```python
from build123d import *

# Parameters (mm, degrees)
IZIM1_R                     = 4.2
Y_KSEKLIK_EKSTR_ZYON1_DEPTH = 12
Y_KSEKLIK_EKSTR_ZYON2_DEPTH = 48
Y_KSEKLIK_EKSTR_ZYON3_DEPTH = 3.5


with BuildPart() as part:
    # Çizim1 → Yükseklik-Ekstrüzyon1 (new body)
    with BuildSketch(Plane.XY):
        with BuildLine():
            Line((-17.5, 16), (17.5, 16))
            ThreePointArc((17.5, 16), (24.571067812, 13.071067812), (27.5, 6))
            Line((27.5, 6), (27.5, -16))
            Line((27.5, -16), (-27.5, -16))
            Line((-27.5, -16), (-27.5, 6))
            ThreePointArc((-27.5, 6), (-24.571067812, 13.071067812), (-17.5, 16))
        make_face()
        with Locations((-20, 6)):
            Circle(IZIM1_R, mode=Mode.SUBTRACT)
        with Locations((20, 6)):
            Circle(IZIM1_R, mode=Mode.SUBTRACT)
    extrude(amount=Y_KSEKLIK_EKSTR_ZYON1_DEPTH)

    # Çizim2 → Yükseklik-Ekstrüzyon2 (add)
    with BuildSketch(Plane.XY.offset(12)):
        with BuildLine():
            Line((-27.5, -16), (-12, -16))
            Line((-12, -16), (-12, -8))
            Line((-12, -8), (12, -8))
            Line((12, -8), (12, -16))
            Line((12, -16), (27.5, -16))
            Line((27.5, -16), (27.5, -4))
            ThreePointArc((27.5, -4), (26.328427125, -1.171572875), (23.5, 0))
            Line((23.5, 0), (-23.5, 0))
            ThreePointArc((-23.5, 0), (-26.328427125, -1.171572875), (-27.5, -4))
            Line((-27.5, -4), (-27.5, -16))
        make_face()
    extrude(amount=Y_KSEKLIK_EKSTR_ZYON2_DEPTH)

    # Çizim3 → Yükseklik-Ekstrüzyon3 (add, symmetric)
    with BuildSketch(Plane(origin=(0, 0, 0), x_dir=(0, 0, -1), z_dir=(1, 0, 0))):
        Polygon((-12, 16), (-47, 0), (-12, 0), align=None)
    extrude(amount=Y_KSEKLIK_EKSTR_ZYON3_DEPTH, both=True)


solid = part.part
```
Can you work these out from the model? Positions are in its coordinate system, mm. A direction names the side the tool comes from. Round coordinates to 2 decimals unless told otherwise and drop trailing zeros. Loops run counter-clockwise (first coordinate to the right, second up) from the corner with the lowest first, then second, coordinate; pieces in that order, holes last. Notation, with made-up numbers: M -4.5,-39.75 L -0.5,-39.75 A22 ccw -0.5,-16.75 Z; hole C 1,52.25 d8. An arc over 180 degrees is marked long. Answer as a JSON object with one key per item and string values. Group by question number.
Q1. Will these pins go through, and if not, where does the flat tip stop? pin 1 (17.5 mm diameter, centred on y = 9.5, z = 30.5, fed in from -X); pin 2 (5 mm diameter, centred on y = 8.5, z = 24.5, fed in from +X); pin 3 (12 mm diameter, centred on y = 3, z = 52.5, fed in from -X); pin 4 (5 mm diameter, centred on x = 20, y = 6, fed in from +Z).
Q2. Please list where these lines run through material, in increasing order: L1, parallel to Z at x = 1.5, y = -9; L2, parallel to Y at x = 20, z = 4; L3, parallel to Y at x = -8, z = 12.5.
Q3. On a 3-axis mill with a long thin cutter (end or side, diameter ignored), from which of +Z, -Z, +X, -X, +Y, -Y can I reach the whole of each face in a straight line? I mean faces 4 (the flat face through (3.5, 5, 22)), 5 (the flat face through (6, 0, 36)), 6 (the flat face through (-15, 8, 12)), 7 (the flat face through (-12, -12, 36)). Say none if no direction works.
Q4. Imagine slicing it at B-B, the plane x = -20. Please give me the cut outline in (y, z), then the cut area to 3 significant figures.
Q5. Imagine slicing it at A-A, the plane z = 6.5. Please give me the cut outline in (x, y).
Q6. Imagine slicing it at C-C, the plane z = 26. Please give me the cut outline in (x, y), then the cut area to 3 significant figures.
Q7. Imagine slicing it at D-D, the plane y = -2. Please give me the cut outline in (x, z), then the cut area to 3 significant figures.
Q8. We'd pull the mould along X, two halves only. Please class faces 1 (the flat face through (-13, -16, 23)), 2 (the flat face through (12, -12, 36)), 3 (the flat face through (-27.5, -7, 23)): +X half, -X half, draft (parallel to the pull), parting line (faces both ways), or undercut.
Findings:
{
 "1": {"pin 1": "stops at x = -3.5", "pin 2": "stops at x = 3.5", "pin 3": "stops at x = -27.37", "pin 4": "passes through"},
 "2": {"L1": "z = 0 to 12", "L2": "y = -16 to 1.8, 10.2 to 15.68", "L3": "y = -8 to 0"},
 "3": {"face 4": "+Z, +X, +Y", "face 5": "+Z, +Y", "face 6": "+Z, -X, +Y", "face 7": "+Z, -Y"},
 "4": {"outline": "M -16,0 L 1.8,0 L 1.8,12 L 0,12 L 0,60 L -16,60 Z; M 10.2,0 L 15.68,0 L 15.68,12 L 10.2,12 Z", "area": "1,050 mm2"},
 "5": {"outline": "M -27.5,-16 L 27.5,-16 L 27.5,6 A10 ccw 17.5,16 L -17.5,16 A10 ccw -27.5,6 Z; hole C -20,6 d8.4; hole C 20,6 d8.4"},
 "6": {"outline": "M -27.5,-16 L -12,-16 L -12,-8 L 12,-8 L 12,-16 L 27.5,-16 L 27.5,-4 A4 ccw 23.5,0 L 3.5,0 L 3.5,9.6 L -3.5,9.6 L -3.5,0 L -23.5,0 A4 ccw -27.5,-4 Z", "area": "748 mm2"},
 "7": {"outline": "M -27.5,0 L 27.5,0 L 27.5,12 L 26.96,12 L 26.96,60 L -26.96,60 L -26.96,12 L -27.5,12 Z", "area": "3,250 mm2"},
 "8": {"face 1": "draft", "face 2": "undercut", "face 3": "-X half"}
}
